Design review of the part built by this model. Coordinates are the model's own, in mm. A direction names the side the tool comes from. Round coordinates to 2 decimals unless told otherwise and drop trailing zeros. Write each loop counter-clockwise with the first axis right and the second up, starting at its lowest first coordinate (ties: lowest second). Pieces come first, ordered by that corner, then holes. Notation, with made-up numbers: (16.5, 70.25) - (56.5, 70.25) arc R20 cw to (56.5, 93.25) - close; hole circle Ø6 at (31.5, 49.25). An arc over 180 degrees is marked (long way). Use one line per item in the form item = value.
Autodesk Inventor part; units mm, degrees
ref_plane "YZ Plane" through (0, 0, 0) normal (1, 0, 0) x (0, 1, 0)
ref_plane "XZ Plane" through (0, 0, 0) normal (0, 1, 0) x (-1, 0, 0)
ref_plane "XY Plane" through (0, 0, 0) normal (0, 0, 1) x (1, 0, 0)
sketch "스케치1" plane through (0, 0, 0) normal (0, 0, 1) x (1, 0, 0)
  circle A0 centre (0, 0) radius 22
  line L0 (0, 0) -> (0, 18)
  line L1 (-0.15, -20.7995) -> (-0.15, -19.593)
  arc A1 (-0.15, -16.407) -> (-0.15, -19.593) centre (0, -18) ccw
  line L2 (-0.15, -16.407) -> (-0.15, -12.9991)
  arc A2 (0.15, -12.9991) -> (-0.15, -12.9991) centre (0, 0) ccw
  line L3 (0.15, -16.407) -> (0.15, -12.9991)
  arc A3 (0.15, -19.593) -> (0.15, -16.407) centre (0, -18) ccw
  line L4 (0.15, -20.7995) -> (0.15, -19.593)
  circle A4 centre (12, 12) radius 1.6
  circle A5 centre (-18, 0) radius 1.6
  circle A6 centre (-12, 12) radius 1.6
  circle A7 centre (-12, -12) radius 1.6
  circle A8 centre (18, 0) radius 1.6
  circle A9 centre (12, -12) radius 1.6
  circle A10 centre (0, 18) radius 1.6
  circle A11 centre (0, 0) radius 12.5
  circle A12 centre (0, -18) radius 1.6
  point P0 (0.15, -19.593)
  dimension "d0" = 44
  dimension "d1" = 18
extrude "돌출1" add sketch "스케치1" along normal blind 4 contours A0 | A2 L3 A12 L2 | A10 | A11 | A3 A12 A1 | A4 | A5 | A6 | A7 | A8 | A9
sketch "스케치2" plane through (0, 0, 4) normal (0, 0, 1) x (1, 0, 0)
  circle A0 centre (0, 0) radius 22
  circle A1 centre (0, 0) radius 22
  line L0 (0, -22) -> (0, 58)
  line L1 (22, 0) -> (22, 53.7157)
  line L2 (16.1421, 67.8579) -> (-6.2843, 90.2843)
  line L3 (22, 62) -> (53.7157, 62) construction
  line L4 (-6.2843, 90.2843) -> (-37.397, 59.1716)
  line L5 (-22, 0) -> (-22, 35.4903)
  line L6 (-27.8579, 49.6325) -> (-37.397, 59.1716)
  arc A2 (-22, 35.4903) -> (-27.8579, 49.6325) centre (-42, 35.4903) ccw
  arc A3 (22, 53.7157) -> (16.1421, 67.8579) centre (2, 53.7157) ccw
  point P0 (-22, 43.7746)
  dimension "d9" = 80
  dimension "d46" = 62
  dimension "d48" = 135
  dimension "d50" = 40
  dimension "d57" = 20
  dimension "d92" = 44
sketch "스케치4" plane through (0, 0, 4) normal (0, 0, 1) x (1, 0, 0)
  circle A0 centre (0, 0) radius 14
  dimension "d32" = 28
extrude "돌출4" cut sketch "스케치4" against normal blind 4
sketch "스케치5" plane through (0, 0, 4) normal (0, 0, 1) x (1, 0, 0)
  line L0 (-0.0007, 55) -> (-0.0007, 47)
  line L1 (-0.0007, 47) -> (10.9993, 47)
  line L2 (-0.0007, 47) -> (-11.0007, 47)
  line L3 (-0.0007, 47) -> (-0.0007, 27)
  line L4 (-12.6007, 43.8) -> (-1.6007, 29.1333)
  line L5 (12.5993, 43.8) -> (1.5993, 29.1333)
  line L6 (11.3993, 37.2) -> (4.7993, 28.4)
  line L7 (6.3993, 25.2) -> (12.9993, 25.2)
  line L8 (14.9993, 27.2) -> (14.9993, 36)
  arc A0 (-11.0007, 47) -> (-12.6007, 43.8) centre (-11.0007, 45) ccw
  arc A1 (-1.6007, 29.1333) -> (1.5993, 29.1333) centre (-0.0007, 30.3333) ccw
  arc A2 (12.5993, 43.8) -> (10.9993, 47) centre (10.9993, 45) ccw
  arc A3 (14.9993, 36) -> (11.3993, 37.2) centre (12.9993, 36) ccw
  arc A4 (12.9993, 25.2) -> (14.9993, 27.2) centre (12.9993, 27.2) ccw
  arc A5 (4.7993, 28.4) -> (6.3993, 25.2) centre (6.3993, 27.2) ccw
  line L9 (-11.4007, 37.2) -> (-4.8007, 28.4)
  line L10 (-6.4007, 25.2) -> (-13.0007, 25.2)
  line L11 (-15.0007, 27.2) -> (-15.0007, 36)
  arc A6 (-11.4007, 37.2) -> (-15.0007, 36) centre (-13.0007, 36) ccw
  arc A7 (-15.0007, 27.2) -> (-13.0007, 25.2) centre (-13.0007, 27.2) ccw
  arc A8 (-6.4007, 25.2) -> (-4.8007, 28.4) centre (-6.4007, 27.2) ccw
  point P0 (0, 0)
  point P1 (14.9993, 47)
  point P2 (-15.0007, 47)
  point P3 (14.9993, 42)
  dimension "d35" = 8
  dimension "d36" = 15
  dimension "d37" = 15
  dimension "d38" = 20
  dimension "d39" = 5
  dimension "d41" = 2
extrude "돌출7" add sketch "스케치2" against normal blind 4 contours L5 A2 L6 L4 L2 A3 L1 A0
extrude "돌출8" cut sketch "스케치5" against normal blind 4
extrude "돌출9" cut sketch "스케치1" along normal blind 4 contours A10 | A3 A12 A1 | A4 | A5 | A6 | A7 | A8 | A9
sketch "스케치9" plane through (0, 0, 4) normal (0, 0, 1) x (1, 0, 0)
  circle A0 centre (-12, 12) radius 1.6
  circle A1 centre (12, -12) radius 1.6
  circle A2 centre (0, -18) radius 1.6
  circle A3 centre (0, 18) radius 1.6
  circle A4 centre (-18, 0) radius 1.6
  circle A5 centre (18, 0) radius 1.6
  circle A6 centre (-12, -12) radius 1.6
  circle A7 centre (12, 12) radius 1.6
  line L0 (4.7993, 28.4) -> (11.3993, 37.2)
  arc A8 (14.9993, 36) -> (11.3993, 37.2) centre (12.9993, 36) ccw
  line L1 (14.9993, 36) -> (14.9993, 27.2)
  arc A9 (12.9993, 25.2) -> (14.9993, 27.2) centre (12.9993, 27.2) ccw
  line L2 (12.9993, 25.2) -> (6.3993, 25.2)
  arc A10 (4.7993, 28.4) -> (6.3993, 25.2) centre (6.3993, 27.2) ccw
  arc A11 (-6.4007, 25.2) -> (-4.8007, 28.4) centre (-6.4007, 27.2) ccw
  line L3 (-6.4007, 25.2) -> (-13.0007, 25.2)
  arc A12 (-15.0007, 27.2) -> (-13.0007, 25.2) centre (-13.0007, 27.2) ccw
  line L4 (-15.0007, 27.2) -> (-15.0007, 36)
  arc A13 (-11.4007, 37.2) -> (-15.0007, 36) centre (-13.0007, 36) ccw
  line L5 (-11.4007, 37.2) -> (-4.8007, 28.4)
  line L6 (12.5993, 43.8) -> (1.5993, 29.1333)
  arc A14 (-1.6007, 29.1333) -> (1.5993, 29.1333) centre (-0.0007, 30.3333) ccw
  line L7 (-1.6007, 29.1333) -> (-12.6007, 43.8)
  arc A15 (-11.0007, 47) -> (-12.6007, 43.8) centre (-11.0007, 45) ccw
  line L8 (-11.0007, 47) -> (10.9993, 47)
  arc A16 (12.5993, 43.8) -> (10.9993, 47) centre (10.9993, 45) ccw
  circle A17 centre (0, 0) radius 14
  arc A18 (-22, 0) -> (22, 0) centre (0, 0) ccw
  line L9 (22, 0) -> (22, 53.7157)
  arc A19 (22, 53.7157) -> (16.1421, 67.8579) centre (2, 53.7157) ccw
  line L10 (16.1421, 67.8579) -> (-6.2843, 90.2843)
  line L11 (-6.2843, 90.2843) -> (-37.397, 59.1716)
  line L12 (-37.397, 59.1716) -> (-27.8579, 49.6325)
  arc A20 (-22, 35.4903) -> (-27.8579, 49.6325) centre (-42, 35.4903) ccw
  line L13 (-22, 35.4903) -> (-22, 0)
  circle A21 centre (-29.2652, 60.9393) radius 1.6
  circle A22 centre (-22.1942, 68.0104) radius 1.6
  circle A23 centre (-15.1231, 75.0815) radius 1.6
  circle A24 centre (-8.052, 82.1525) radius 1.6
  dimension "d73" = 3.2
  dimension "d74" = 3.2
  dimension "d76" = 3.2
  dimension "d77" = 3.2
  dimension "d78" = 4.5
  dimension "d79" = 4.5
  dimension "d81" = 4.5
  dimension "d82" = 4.5
  dimension "d83" = 10
  dimension "d85" = 10
  dimension "d88" = 7
  dimension "d91" = 7
extrude "돌출10" cut sketch "스케치9" against normal blind 10 contours A21 | A22 | A23 | A24
sketch "스케치10" plane through (0, 0, 4) normal (0, 0, 1) x (1, 0, 0)
  circle A0 centre (-15.1231, 75.0815) radius 1.6
  circle A1 centre (-22.1942, 68.0104) radius 1.6
  circle A2 centre (-8.052, 82.1525) radius 1.6
  circle A3 centre (-29.2652, 60.9393) radius 1.6
  circle A4 centre (-12, 12) radius 1.6
  circle A5 centre (12, -12) radius 1.6
  circle A6 centre (0, -18) radius 1.6
  circle A7 centre (0, 18) radius 1.6
  circle A8 centre (-18, 0) radius 1.6
  circle A9 centre (18, 0) radius 1.6
  circle A10 centre (-12, -12) radius 1.6
  circle A11 centre (12, 12) radius 1.6
  line L0 (4.7993, 28.4) -> (11.3993, 37.2)
  arc A12 (14.9993, 36) -> (11.3993, 37.2) centre (12.9993, 36) ccw
  line L1 (14.9993, 36) -> (14.9993, 27.2)
  arc A13 (12.9993, 25.2) -> (14.9993, 27.2) centre (12.9993, 27.2) ccw
  line L2 (12.9993, 25.2) -> (6.3993, 25.2)
  arc A14 (4.7993, 28.4) -> (6.3993, 25.2) centre (6.3993, 27.2) ccw
  arc A15 (-6.4007, 25.2) -> (-4.8007, 28.4) centre (-6.4007, 27.2) ccw
  line L3 (-6.4007, 25.2) -> (-13.0007, 25.2)
  arc A16 (-15.0007, 27.2) -> (-13.0007, 25.2) centre (-13.0007, 27.2) ccw
  line L4 (-15.0007, 27.2) -> (-15.0007, 36)
  arc A17 (-11.4007, 37.2) -> (-15.0007, 36) centre (-13.0007, 36) ccw
  line L5 (-11.4007, 37.2) -> (-4.8007, 28.4)
  line L6 (12.5993, 43.8) -> (1.5993, 29.1333)
  arc A18 (-1.6007, 29.1333) -> (1.5993, 29.1333) centre (-0.0007, 30.3333) ccw
  line L7 (-1.6007, 29.1333) -> (-12.6007, 43.8)
  arc A19 (-11.0007, 47) -> (-12.6007, 43.8) centre (-11.0007, 45) ccw
  line L8 (-11.0007, 47) -> (10.9993, 47)
  arc A20 (12.5993, 43.8) -> (10.9993, 47) centre (10.9993, 45) ccw
  circle A21 centre (0, 0) radius 14
  arc A22 (-22, 0) -> (22, 0) centre (0, 0) ccw
  line L9 (22, 0) -> (22, 53.7157)
  arc A23 (22, 53.7157) -> (16.1421, 67.8579) centre (2, 53.7157) ccw
  line L10 (16.1421, 67.8579) -> (-6.2843, 90.2843)
  line L11 (-6.2843, 90.2843) -> (-37.397, 59.1716)
  line L12 (-37.397, 59.1716) -> (-27.8579, 49.6325)
  arc A24 (-22, 35.4903) -> (-27.8579, 49.6325) centre (-42, 35.4903) ccw
  line L13 (-22, 35.4903) -> (-22, 0)
  line L14 (-6.2843, 90.2843) -> (16.1421, 67.8579)
  line L15 (-6.2843, 90.2843) -> (-13.3553, 97.3553)
  line L16 (-13.3553, 97.3553) -> (-44.468, 66.2426)
  line L17 (-44.468, 66.2426) -> (-37.397, 59.1716)
  line L18 (-14.7696, 92.4056) -> (-39.5183, 67.6569)
  line L19 (-6.2843, 90.2843) -> (-37.397, 59.1716)
  line L20 (-39.5183, 67.6569) -> (-35.9828, 64.1213)
  line L21 (-35.9828, 64.1213) -> (-11.234, 88.8701)
  line L22 (-11.234, 88.8701) -> (-14.7696, 92.4056)
  point P0 (-37.397, 59.1716)
  dimension "d93" = 10
  dimension "d95" = 5
  dimension "d96" = 35
  dimension "d97" = 2.5
  dimension "d99" = 4.5
extrude "돌출11" add sketch "스케치10" against normal blind 4 contours L17 L16 L15 L11
fillet "모깎기1" radius 2 2 edges at (-13.3553, 97.3553, 2) (-44.468, 66.2426, 2)
sketch "스케치11" plane through (0, 0, 4) normal (0, 0, 1) x (1, 0, 0)
  arc A0 (-43.0538, 67.6569) -> (-43.0538, 64.8284) centre (-41.6396, 66.2426) ccw
  line L0 (-43.0538, 64.8284) -> (-27.8579, 49.6325)
  arc A1 (-22, 35.4903) -> (-27.8579, 49.6325) centre (-42, 35.4903) ccw
  line L1 (-22, 35.4903) -> (-22, 0)
  arc A2 (-22, 0) -> (22, 0) centre (0, 0) ccw
  line L2 (22, 0) -> (22, 53.7157)
  arc A3 (22, 53.7157) -> (16.1421, 67.8579) centre (2, 53.7157) ccw
  line L3 (16.1421, 67.8579) -> (-11.9411, 95.9411)
  arc A4 (-11.9411, 95.9411) -> (-14.7696, 95.9411) centre (-13.3553, 94.5269) ccw
  line L4 (-14.7696, 95.9411) -> (-43.0538, 67.6569)
  line L5 (-35.9828, 64.1213) -> (-39.5183, 67.6569)
  line L6 (-39.5183, 67.6569) -> (-14.7696, 92.4056)
  line L7 (-14.7696, 92.4056) -> (-11.234, 88.8701)
  line L8 (-11.234, 88.8701) -> (-35.9828, 64.1213)
  circle A5 centre (-15.1231, 75.0815) radius 1.6
  circle A6 centre (-22.1942, 68.0104) radius 1.6
  circle A7 centre (-8.052, 82.1525) radius 1.6
  circle A8 centre (-29.2652, 60.9393) radius 1.6
  circle A9 centre (-12, 12) radius 1.6
  circle A10 centre (12, -12) radius 1.6
  circle A11 centre (0, -18) radius 1.6
  circle A12 centre (0, 18) radius 1.6
  circle A13 centre (-18, 0) radius 1.6
  circle A14 centre (18, 0) radius 1.6
  circle A15 centre (-12, -12) radius 1.6
  circle A16 centre (12, 12) radius 1.6
  arc A17 (4.7993, 28.4) -> (6.3993, 25.2) centre (6.3993, 27.2) ccw
  line L9 (4.7993, 28.4) -> (11.3993, 37.2)
  arc A18 (14.9993, 36) -> (11.3993, 37.2) centre (12.9993, 36) ccw
  line L10 (14.9993, 36) -> (14.9993, 27.2)
  arc A19 (12.9993, 25.2) -> (14.9993, 27.2) centre (12.9993, 27.2) ccw
  line L11 (12.9993, 25.2) -> (6.3993, 25.2)
  arc A20 (-6.4007, 25.2) -> (-4.8007, 28.4) centre (-6.4007, 27.2) ccw
  line L12 (-6.4007, 25.2) -> (-13.0007, 25.2)
  arc A21 (-15.0007, 27.2) -> (-13.0007, 25.2) centre (-13.0007, 27.2) ccw
  line L13 (-15.0007, 27.2) -> (-15.0007, 36)
  arc A22 (-11.4007, 37.2) -> (-15.0007, 36) centre (-13.0007, 36) ccw
  line L14 (-11.4007, 37.2) -> (-4.8007, 28.4)
  line L15 (-11.0007, 47) -> (10.9993, 47)
  arc A23 (12.5993, 43.8) -> (10.9993, 47) centre (10.9993, 45) ccw
  line L16 (12.5993, 43.8) -> (1.5993, 29.1333)
  arc A24 (-1.6007, 29.1333) -> (1.5993, 29.1333) centre (-0.0007, 30.3333) ccw
  line L17 (-1.6007, 29.1333) -> (-12.6007, 43.8)
  arc A25 (-11.0007, 47) -> (-12.6007, 43.8) centre (-11.0007, 45) ccw
  circle A26 centre (0, 0) radius 14
  arc A27 (46.1675, 71.3111) -> (47.7675, 68.1111) centre (47.7675, 70.1111) ccw
  line L18 (46.1675, 71.3111) -> (52.7675, 80.1111)
  arc A28 (56.3675, 78.9111) -> (52.7675, 80.1111) centre (54.3675, 78.9111) ccw
  line L19 (56.3675, 78.9111) -> (56.3675, 70.1111)
  arc A29 (54.3675, 68.1111) -> (56.3675, 70.1111) centre (54.3675, 70.1111) ccw
  line L20 (54.3675, 68.1111) -> (47.7675, 68.1111)
  arc A30 (34.9675, 68.1111) -> (36.5675, 71.3111) centre (34.9675, 70.1111) ccw
  line L21 (34.9675, 68.1111) -> (28.3675, 68.1111)
  arc A31 (26.3675, 70.1111) -> (28.3675, 68.1111) centre (28.3675, 70.1111) ccw
  line L22 (26.3675, 70.1111) -> (26.3675, 78.9111)
  arc A32 (29.9675, 80.1111) -> (26.3675, 78.9111) centre (28.3675, 78.9111) ccw
  line L23 (29.9675, 80.1111) -> (36.5675, 71.3111)
  line L24 (30.3675, 89.9111) -> (52.3675, 89.9111)
  arc A33 (53.9675, 86.7111) -> (52.3675, 89.9111) centre (52.3675, 87.9111) ccw
  line L25 (53.9675, 86.7111) -> (42.9675, 72.0445)
  arc A34 (39.7675, 72.0445) -> (42.9675, 72.0445) centre (41.3675, 73.2445) ccw
  line L26 (39.7675, 72.0445) -> (28.7675, 86.7111)
  arc A35 (30.3675, 89.9111) -> (28.7675, 86.7111) centre (30.3675, 87.9111) ccw
  line L27 (-43.0538, 64.8284) -> (-27.8579, 49.6325)
  line L28 (16.1421, 67.8579) -> (-11.9411, 95.9411)
  line L29 (-11.0007, 47) -> (10.9993, 47)
  line L30 (-0.0007, 47) -> (-0.0007, 52)
  line L31 (22, 53.7157) -> (22, 0)
  arc A36 (-22, 35.4903) -> (-27.8579, 49.6325) centre (-42, 35.4903) ccw
  line L32 (-27.8579, 49.6325) -> (3.2548, 80.7452)
  line L33 (-22.0662, 55.4241) -> (-0.0007, 55.4241)
  line L34 (-0.0007, 55.4241) -> (-0.0007, 77.4896)
  dimension "d103" = 5
  dimension "d104" = 22.0655
extrude "돌출12" cut sketch "스케치11" against normal blind 10 contours L32 L34 L33
fillet "모깎기2" radius 2 3 edges at (-22.0662, 55.4241, 2) (-0.0007, 77.4896, 2) (-0.0007, 55.4241, 2)
properties part number "조인트3힌지사이드_4T" material "알루미늄 6061"
Q1. For P1, Ø2.5, axis at x = 18, y = 0, coming from the -Z side; P2, Ø2, axis at y = 32, z = 2, coming from the -X side; P3, Ø2, axis at y = 73.5, z = 0.5, coming from the +X side; P4, Ø2, axis at x = -9, z = 3, coming from the +Y side, all flat-tipped, find the tip position at first contact; note any pin that passes through.
Calculated:
P1 = through
P2 = -22
P3 = 11.5
P4 = 94
Q2. We need section C-C on y = 48.5. Write out the cut boundary in (x, z), then the cut area to 3 significant figures.
Calculated:
outline = (-26.81, 0) - (22, 0) - (22, 4) - (-26.81, 4) - close
area = 195 mm2
Q3. To check wall thickness, follow line 1 along X through (y, z) = (75, 0.7); line 2 along Y through (x, z) = (-30, 2.8); line 3 along Y through (x, z) = (-18, 2.35) (3 decimals). State the ranges of each line that lie inside material, in increasing order. Write a range as from..to.
Calculated:
line_1 = -35.71..-32.18, -25.1..-16.72, -13.53..9
line_2 = 51.77..59.52, 62.36..70.1, 77.18..80.71
line_3 = -12.649..-1.6, 1.6..55.575, 59.49..82.104, 89.175..92.711
Q4. We need section B-B on x = -34. Write out the cut boundary in (y, z).
Calculated:
outline = (55.77, 0) - (66.1, 0) - (66.1, 4) - (55.77, 4) - close; (73.18, 0) - (76.71, 0) - (76.71, 4) - (73.18, 4) - close
Q5. Draft analysis for pull direction X (two halves, no side actions). For faces 1 (the flat face through (2, 82, 2)), 2 (the flat face through (-4, 51, 4)), 3 (the flat face through (-26.971, 80.204, 2.028)), state which applies: released by +X, released by -X, zero draft, split by the parting line, or undercut.
Calculated:
face_1 = released by +X
face_2 = zero draft
face_3 = undercut
Q6. We need section A-A on y = 18. Write out the cut boundary in (x, z), then the cut area to 3 significant figures.
Calculated:
outline = (-22, 0) - (-1.6, 0) - (-1.6, 4) - (-22, 4) - close; (1.6, 0) - (22, 0) - (22, 4) - (1.6, 4) - close
area = 163 mm2
Q7. Machinability: for faces 4 (the flat face through (-35.562, 57.337, 2.028)), 5 (the flat face through (7.2, 36.6, 2)), which of the approach directions +Z, -Z, +X, -X, +Y, -Y give a long, thin tool a straight path to every point of the face, cutting with its end or side? Answer none if there is none.
Calculated:
face_4 = +Z, -Z, -X, -Y
face_5 = +Z, -Z
